Can you work these out from the model? Positions are in its coordinate system, mm. A direction names the side the tool comes from. Coordinates: 2 decimals unless noted, no trailing zeros. Write each loop counter-clockwise with the first axis right and the second up, starting at its lowest first coordinate (ties: lowest second). Pieces come first, ordered by that corner, then holes. Notation, with made-up numbers: (-13.5, -25.5) -> (9.5, -25.5) arc R30 cw to (9.5, 1.5) -> close; hole circle Ø8 at (88, 73). An arc over 180 degrees is marked (long way). Use one line per item in the form item = value.
```python
from build123d import *

# Parameters (mm, degrees)
F0_R        = 6.2865
F1_DEPTH    = 25.4
F2_R        = 4.7625
F3_DEPTH    = 9.525
F4_R        = 2.0955
F5_DEPTH    = 6.35
F5_FACE_R   = 4.7625
F5_FACE_R_2 = 2.0955
F6_DEPTH    = 3.175


with BuildPart() as f1:
    # F0 (on Top) → F1 (new body)
    with BuildSketch(Plane.XY):
        with BuildLine():
            Line((9.525, -9.525), (9.525, 9.525))
            Line((9.525, 9.525), (0, 9.525))
            ThreePointArc((0, 9.525), (-6.735192, 6.735192), (-9.525, 0))
            ThreePointArc((-9.525, 0), (-6.735192, -6.735192), (0, -9.525))
            Line((0, -9.525), (9.525, -9.525))
        make_face()
        Circle(F0_R, mode=Mode.SUBTRACT)
    extrude(amount=F1_DEPTH)

    # F2 (on face) → F3 (join)
    with BuildSketch(Plane.YZ.offset(9.525)):
        with BuildLine():
            Line((-9.525, 25.4), (-20.955, 25.4))
            ThreePointArc((-20.955, 25.4), (-33.655, 12.7), (-20.955, 0))
            Line((-20.955, 0), (-9.525, 0))
            Line((-9.525, 0), (-9.525, 25.4))
        make_face()
        with Locations((-20.955, 12.7)):
            Circle(F2_R, mode=Mode.SUBTRACT)
    extrude(amount=-F3_DEPTH)

    # F4 (on face) → F5 (join)
    with BuildSketch(Plane.YZ.offset(9.525)):
        with BuildLine():
            Line((13.335, 25.4), (9.525, 25.4))
            Line((9.525, 25.4), (9.525, 0))
            Line((9.525, 0), (13.335, 0))
            ThreePointArc((13.335, 0), (17.825128, 1.859872), (19.685, 6.35))
            Line((19.685, 6.35), (19.685, 19.05))
            ThreePointArc((19.685, 19.05), (17.825128, 23.540128), (13.335, 25.4))
        make_face()
        with Locations((14.605, 12.7)):
            Circle(F4_R, mode=Mode.SUBTRACT)
    extrude(amount=-F5_DEPTH)

    # F5_face (on face) → F6 (join)
    with BuildSketch(Plane(origin=(9.525, -5.370405, 12.7), x_dir=(0, 1, 0), z_dir=(1, 0, 0))):
        with BuildLine():
            ThreePointArc((-15.584595, 12.7), (-28.284595, 0), (-15.584595, -12.7))
            Line((-15.584595, -12.7), (18.705405, -12.7))
            ThreePointArc((18.705405, -12.7), (23.195534, -10.840128), (25.055405, -6.35))
            Line((25.055405, -6.35), (25.055405, 6.35))
            ThreePointArc((25.055405, 6.35), (23.195534, 10.840128), (18.705405, 12.7))
            Line((18.705405, 12.7), (-15.584595, 12.7))
        make_face()
        with Locations((-15.584595, 0)):
            Circle(F5_FACE_R, mode=Mode.SUBTRACT)
        with Locations((19.975405, 0)):
            Circle(F5_FACE_R_2, mode=Mode.SUBTRACT)
    extrude(amount=F6_DEPTH)


solid = f1.part
```
Q1. Suppose I cut it at C-C (y = 16). Write out the boundary of the cut face in (x, z) (3 decimals), then the cut area to 3 significant figures.
Return value:
outline = (3.175, 0.586) -> (12.7, 0.586) -> (12.7, 11.136) -> (3.175, 11.136) -> close; (3.175, 14.264) -> (12.7, 14.264) -> (12.7, 24.814) -> (3.175, 24.814) -> close
area = 201 mm2
Q2. For faces 1 (the flat face through (3.175, 12, 13)), 2 (the flat face through (0, -16, 10)), 3 (the flat face through (8, 19.685, 13)), which set-ups out of +Z, -Z, +X, -X, +Y, -Y let a thin tool reach every point of the face, with its end or its side?
Return value:
face_1 = +Z, -Z, -X, +Y
face_2 = +Z, -Z, -X, -Y
face_3 = +Z, -Z, +X, -X, +Y
Q3. If I drill on line 1 (Y direction, x = 1, z = 12.25) (3 decimals); line 2 (X direction, y = -24, z = 18.5); line 3 (Y direction, x = 11, z = 11.5) (3 decimals), over which ranges is the centre line in solid material (lowest first)? Write a range as from..to.
Return value:
line_1 = -33.647..-25.696, -16.214..-6.206, 6.206..9.525
line_2 = 0..12.7
line_3 = -33.598..-25.564, -16.346..12.887, 16.323..19.685
Q4. Will these pins go through, and if not, where does the flat tip stop? pin 1 (10 mm diameter, centred on y = -15, z = 8, fed in from -X); pin 2 (2 mm diameter, centred on y = -5.5, z = 23, fed in from -X) (3 decimals); pin 3 (2.5 mm diameter, centred on y = 14.605, z = 12.7, fed in from +X); pin 4 (7 mm diameter, centred on y = 16.5, z = 4.5, fed in from -X) (3 decimals).
Return value:
pin_1 = 0
pin_2 = -8.395
pin_3 = through
pin_4 = 3.175
Q5. Suppose I cut it at A-A (z = 12.7). Give the number of separate pieces and of enclosed holes in the cut face, then the cut area to 3 significant figures.
Return value:
separate_pieces = 3
enclosed_holes = 1
area = 503 mm2
Q6. Thinking about a two-plate mould opening in Z: for faces 4 (the cylindrical face through (6.394, 17.775, 1.811)), 5 (the cylindrical face through (7.87, 15.73, 14.47)), 6 (the cylindrical face through (6.261, -16.556, 10.876)), 7 (the flat face through (12.7, -7, 13)), which applies, released by +Z, released by -Z, zero draft, split by the parting line, or undercut?
Return value:
face_4 = released by -Z
face_5 = undercut
face_6 = undercut
face_7 = zero draft
